```python
from build123d import *

# Parameters (mm, degrees)
BOSS_EXTRUDE1_DEPTH = 19
SKETCH2_R           = 1.905
CUT_EXTRUDE1_DEPTH  = 10.16
CHAMFER1_SIZE       = 1.016
CHAMFER2_SIZE       = 0.254
CHAMFER3_SIZE       = 1.016


with BuildPart() as part:
    # Sketch1 → Boss-Extrude1 (new body)
    with BuildSketch(Plane(origin=(0, 0, 0), x_dir=(0, 0, -1), z_dir=(1, 0, 0))):
        with BuildLine():
            Line((6.25, -13.87), (-25.5, -13.87))
            Line((-25.5, -13.87), (-25.5, 38))
            Line((-25.5, 38), (25.5, 38))
            Line((25.5, 38), (25.5, 24.08))
            Line((25.5, 24.08), (-6.25, 24.08))
            ThreePointArc((-6.25, 24.08), (-11.33, 19), (-6.25, 13.92))
            Line((-6.25, 13.92), (25.5, 13.92))
            Line((25.5, 13.92), (25.5, -38))
            Line((25.5, -38), (-25.5, -38))
            Line((-25.5, -38), (-25.5, -24.03))
            Line((-25.5, -24.03), (6.25, -24.03))
            ThreePointArc((6.25, -24.03), (11.33, -18.95), (6.25, -13.87))
        make_face()
    extrude(amount=BOSS_EXTRUDE1_DEPTH)

    # Sketch2 → Cut-Extrude1 (cut)
    with BuildSketch(Plane.XZ.offset(38)):
        with Locations(Location((9.5, 0, 0), (0, 0, 270))):
            Circle(SKETCH2_R)
    cut_extrude1 = extrude(amount=-CUT_EXTRUDE1_DEPTH, mode=Mode.SUBTRACT)

    # Chamfer1
    chamfer1_edges = [part.edges().sort_by_distance(p)[0] for p in [
        (9.5, -38, 1.905),
    ]]
    chamfer(chamfer1_edges, length=CHAMFER1_SIZE)

    # Chamfer2
    chamfer2_edges = [part.edges().sort_by_distance(p)[0] for p in [
        (19, -18.95, -11.33),
        (0, 12.065, 25.5),
        (0, 38, 0),
        (0, 31.04, -25.5),
        (0, 24.08, -9.625),
        (19, -24.03, 9.625),
        (0, 19, 11.33),
        (0, 13.92, -9.625),
        (0, -12.04, -25.5),
        (0, -38, 0),
        (0, -31.015, 25.5),
        (0, -24.03, 9.625),
        (0, -18.95, -11.33),
        (0, -13.87, 9.625),
        (19, -31.015, 25.5),
        (9.5, -13.87, 25.5),
        (9.5, 38, 25.5),
        (9.5, 38, -25.5),
        (9.5, 24.08, -25.5),
        (9.5, 13.92, -25.5),
        (9.5, -38, -25.5),
        (9.5, -38, 25.5),
        (9.5, -24.03, 25.5),
        (19, -38, 0),
        (19, -12.04, -25.5),
        (19, 13.92, -9.625),
        (19, 19, 11.33),
        (19, 24.08, -9.625),
        (19, 31.04, -25.5),
        (19, 38, 0),
        (19, -13.87, 9.625),
        (19, 12.065, 25.5),
    ]]
    chamfer(chamfer2_edges, length=CHAMFER2_SIZE)

    # Mirror3: Cut-Extrude1 across plane
    add(cut_extrude1.mirror(Plane.ZX), mode=Mode.SUBTRACT)

    # Chamfer3
    chamfer3_edges = [part.edges().sort_by_distance(p)[0] for p in [
        (9.5, 38, 1.905),
    ]]
    chamfer(chamfer3_edges, length=CHAMFER3_SIZE)


solid = part.part
```
Source: CAD feature listing. Evaluate the final solid. Frame: model axes, mm. A direction names the side the tool comes from. Coordinates: 2 decimals unless noted, no trailing zeros. Loops run counter-clockwise (first coordinate to the right, second up) from the corner with the lowest first, then second, coordinate; pieces in that order, holes last. Notation, with made-up numbers: M 48,0 L 83,0 A23 cw 83,9 Z; hole C 81.25,41.25 d8. An arc over 180 degrees is marked long. Put each result on its own line as item: value. Start each with the question number.
1) Contact query for flat-ended pins moving along their axis: pin 1 Ø4 at (x, z) = (10, -0.5) entering from -Y; pin 2 Ø2.5 at (x, z) = (9.5, 0) entering from -Y; pin 3 Ø1.1 at (x, z) = (9.5, 0) entering from +Y. Output: stop coordinate, or through.
2) Cut plane A-A on z = 21.5. Return the cut outline in (x, y).
3) Cut plane D-D on z = 0. Give the number of separate pieces and of enclosed holes in the cut face, then the cut area to 3 significant figures.
4) Reachability of faces 4 (the face through (11.39, -32.48, 0.25)), 5 (the face through (9, 13.92, -9)), 6 (the face through (9, -13.87, 9)) from +Z, -Z, +X, -X, +Y, -Y: full face, straight path, thin tool, end or side. Return the list, or none.
5) Pull-direction query (Y, two-part tool) for faces 1 (the face through (9, -31, 25.5)), 2 (the face through (10, 27.84, 0)), 3 (the face through (9, 24.08, -10)); classes: pulls with the +Y half, pulls with the -Y half, needs draft (parallel to the pull), parting line crosses it, or undercut.
6) Ray query, L1, parallel to Y at x = 12, z = -3; L2, parallel to Y at x = 15, z = -12.5; L3, parallel to X at y = -30.5, z = 0 (3 decimals). Return the intervals inside material, ascending. Write a range as from..to.
7) Cut plane B-B on y = -18.95. Return the cut outline in (x, z).
The answers:
1. pin 1: stops at y = -37.79
1. pin 2: stops at y = -27.84
1. pin 3: stops at y = 27.84
2. outline: M 0,-37.75 L 0.25,-38 L 18.75,-38 L 19,-37.75 L 19,-24.28 L 18.75,-24.03 L 0.25,-24.03 L 0,-24.28 Z; M 0,-13.62 L 0.25,-13.87 L 18.75,-13.87 L 19,-13.62 L 19,37.75 L 18.75,38 L 0.25,38 L 0,37.75 Z
3. separate pieces: 3
3. enclosed holes: 0
3. area: 978 mm²
4. face 4: -Y
4. face 5: -Z, +X, -X
4. face 6: +Z, +X, -X
5. face 1: needs draft
5. face 2: pulls with the +Y half
5. face 3: undercut
6. L1: y = -38..-24.03, -13.87..13.92, 24.08..38
6. L2: y = -38..13.92, 24.08..38
6. L3: x = 0..7.595, 11.405..19
7. outline: M 0,-25.25 L 0.25,-25.5 L 18.75,-25.5 L 19,-25.25 L 19,-11.58 L 18.75,-11.33 L 0.25,-11.33 L 0,-11.58 Z
